Source: CAD feature listing. Evaluate the final solid. Frame: model axes, mm. Face numbers are marked on the shaded views. Coordinates: 2 decimals unless noted, no trailing zeros. Loops run counter-clockwise (first coordinate to the right, second up) from the corner with the lowest first, then second, coordinate; pieces in that order, holes last. Notation, with made-up numbers: M 26,-12.5 L 52,-12.5 A19 cw 52,17.5 Z; hole C 88.25,24.25 d11. An arc over 180 degrees is marked long. One line per question, with ' | ' between items. Start each with the question number.
1. Mould query, pull axis Y, two halves, no side actions, for the marked faces 1, 2 and 3. Classes: pulls with the +Y half, pulls with the -Y half, needs draft (parallel to the pull), parting line crosses it, or undercut.
2. Section query C-C, the plane y = -17.5. Output: boundary loops of the cut face in (x, z), and give its area (3 significant figures).
3. Pin query (flat end, axial travel): P1, Ø3, axis at x = -1, z = 4, coming from the -Y side; P2, Ø1, axis at y = -7.5, z = 8, coming from the +X side; P3, Ø3, axis at x = -6, z = 1.5, coming from the +Y side. Return the tip coordinate at first contact, or that it passes through.
4. Section query D-D, the plane z = 7.5. Output: boundary loops of the cut face in (x, y), and give its area (3 significant figures).
5. Section query A-A, the plane x = 0. Output: boundary loops of the cut face in (y, z).
6. Ray query, probe 1 along Y at (x, z) = (0, 4.5); probe 2 along Z at (x, y) = (34, -18.5); probe 3 along X at (y, z) = (2, 8). Return the intervals inside material, ascending.
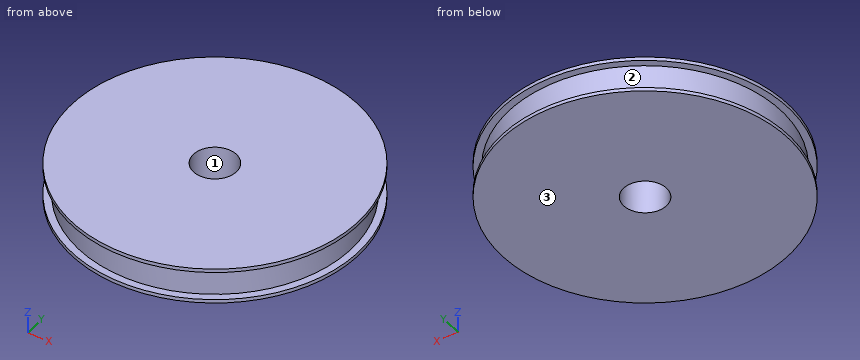
```python
from build123d import *

# Parameters (mm, degrees)
SKETCH1_R           = 40
SKETCH1_R_2         = 38
SKETCH1_R_3         = 6
BOSS_EXTRUDE1_DEPTH = 10
CUT_EXTRUDE1_START  = 1
SKETCH1_3_R         = 40
SKETCH1_3_R_2       = 38
CUT_EXTRUDE1_DEPTH  = 8


with BuildPart() as part:
    # Sketch1 → Boss-Extrude1 (new body)
    # profile 1 of 2: a face of its own
    with BuildSketch(Plane.XY):
        Circle(SKETCH1_R)
        Circle(SKETCH1_R_2, mode=Mode.SUBTRACT)
    # profile 2 of 2: a face of its own
    with BuildSketch(Plane.XY):
        Circle(SKETCH1_R_2)
        Circle(SKETCH1_R_3, mode=Mode.SUBTRACT)
    extrude(amount=BOSS_EXTRUDE1_DEPTH)

    # Sketch1_3 → Cut-Extrude1 (cut)
    with BuildSketch(Plane.XY.offset(CUT_EXTRUDE1_START)):
        Circle(SKETCH1_3_R)
        Circle(SKETCH1_3_R_2, mode=Mode.SUBTRACT)
    extrude(amount=CUT_EXTRUDE1_DEPTH, mode=Mode.SUBTRACT)


solid = part.part
```
Taken from the geometry:
1) face 1: undercut | face 2: parting line crosses it | face 3: needs draft
2) outline: M -35.97,0 L 35.97,0 L 35.97,1 L 33.73,1 L 33.73,9 L 35.97,9 L 35.97,10 L -35.97,10 L -35.97,9 L -33.73,9 L -33.73,1 L -35.97,1 Z | area: 684 mm^2
3) P1: y = -38 | P2: x = 37.35 | P3: y = 39.74
4) outline: C 0,0 d76; hole C 0,0 d12 | area: 4,420 mm^2
5) outline: M -40,0 L -6,0 L -6,10 L -40,10 L -40,9 L -38,9 L -38,1 L -40,1 Z; M 6,0 L 40,0 L 40,1 L 38,1 L 38,9 L 40,9 L 40,10 L 6,10 Z
6) probe 1: -38 to -6, 6 to 38 | probe 2: 0 to 1, 9 to 10 | probe 3: -37.95 to -5.66, 5.66 to 37.95
